from build123d import *

# Parameters (mm, degrees)
SKETCH1_W                 = 23
SKETCH1_H                 = 33
BOSS_EXTRUDE1_DEPTH       = 46
CUT_EXTRUDE1_START        = 12
SKETCH2_W                 = 23
SKETCH2_H                 = 17
CUT_EXTRUDE1_DEPTH        = 26
SKETCH3_R                 = 2.5
CUT_EXTRUDE2_DEPTH        = 6
CUT_EXTRUDE3_START        = -6
SKETCH4_R                 = 2.5
CUT_EXTRUDE3_DEPTH        = 6
CHAMFER1_SIZE             = 6
BOSS_EXTRUDE2_DEPTH       = 26.5
BOSS_EXTRUDE2_DEPTH_BACK  = 23
SKETCH6_W                 = 3
SKETCH6_H                 = 46
F_5_0MM_DOWEL_HOLE1_D     = 5
F_5_0MM_DOWEL_HOLE1_DEPTH = 10
F_5_0MM_DOWEL_HOLE1_TIP   = 1.502151548
SKETCH14_W                = 10
SKETCH14_H                = 10
CUT_EXTRUDE4_DEPTH        = 70.685005561
FILLET1_DEPTH             = 46
FILLET1_START             = 26
FILLET1_2_DEPTH           = 20
FILLET1_3_DEPTH           = 16


with BuildPart() as part:
    # Sketch1 → Boss-Extrude1 (new body)
    with BuildSketch(Plane(origin=(0, 0, 0), x_dir=(1, 0, 0), z_dir=(0, 1, 0))):
        Rectangle(SKETCH1_W, SKETCH1_H)
    extrude(amount=BOSS_EXTRUDE1_DEPTH)

    # Sketch2 → Cut-Extrude1 (cut)
    with BuildSketch(Plane(origin=(0, 0, 0), x_dir=(1, 0, 0), z_dir=(0, 1, 0)).offset(CUT_EXTRUDE1_START)):
        with Locations((0, 8)):
            Rectangle(SKETCH2_W, SKETCH2_H)
    extrude(amount=CUT_EXTRUDE1_DEPTH, mode=Mode.SUBTRACT)

    # Sketch3 → Cut-Extrude2 (cut)
    with BuildSketch(Plane(origin=(0, 46, 0), x_dir=(1, 0, 0), z_dir=(0, 1, 0))):
        with Locations(Location((0, -11.5, 0), (0, 0, 270))):
            Circle(SKETCH3_R)
        with Locations(Location((0, 3.5, 0), (0, 0, 270))):
            Circle(SKETCH3_R)
    extrude(amount=-CUT_EXTRUDE2_DEPTH, mode=Mode.SUBTRACT)

    # Sketch4 → Cut-Extrude3 (cut)
    with BuildSketch(Plane.XZ.offset(CUT_EXTRUDE3_START)):
        with Locations(Location((0, -3.5, 0), (0, 0, 90))):
            Circle(SKETCH4_R)
        with Locations(Location((0, 11.5, 0), (0, 0, 90))):
            Circle(SKETCH4_R)
    extrude(amount=CUT_EXTRUDE3_DEPTH, mode=Mode.SUBTRACT)

    # Chamfer1
    chamfer1_edges = [part.edges().sort_by_distance(p)[0] for p in [
        (11.5, 25, 0.5),
    ]]
    chamfer(chamfer1_edges, length=CHAMFER1_SIZE)

    # Sketch6 → Boss-Extrude2 (add, two sides: drawn at the far end of the back side and taken through both)
    with BuildSketch(Plane(origin=(11.5, 0, 0), x_dir=(0, 0, -1), z_dir=(1, 0, 0)).offset(-BOSS_EXTRUDE2_DEPTH_BACK)):
        with Locations((-18, 23)):
            Rectangle(SKETCH6_W, SKETCH6_H)
    extrude(amount=BOSS_EXTRUDE2_DEPTH + BOSS_EXTRUDE2_DEPTH_BACK)

    # Ø5.0mm Dowel Hole1
    with Locations(Plane(origin=(0, 0, -16.5), x_dir=(-1, 0, 0), z_dir=(0, 0, -1))):
        with Locations((-8, 42), (-8, 8), (8, 8), (8, 42)):
            Hole(F_5_0MM_DOWEL_HOLE1_D / 2, depth=F_5_0MM_DOWEL_HOLE1_DEPTH)
            with Locations((0, 0, -(F_5_0MM_DOWEL_HOLE1_DEPTH + F_5_0MM_DOWEL_HOLE1_TIP / 2))):  # 118° drill point
                Cone(0, F_5_0MM_DOWEL_HOLE1_D / 2, F_5_0MM_DOWEL_HOLE1_TIP, mode=Mode.SUBTRACT)

    # Sketch14 → Cut-Extrude4 (cut, through all)
    with BuildSketch(Plane.XY.offset(19.5)):
        with Locations((23, 21)):
            Rectangle(SKETCH14_W, SKETCH14_H)
    extrude(amount=-CUT_EXTRUDE4_DEPTH, mode=Mode.SUBTRACT)

    # Sketch15 → Cut-Revolve1 (revolve, cut)
    with BuildSketch(Plane(origin=(0, 0, 0), x_dir=(0, 0, -1), z_dir=(1, 0, 0))):
        Polygon((16.5, 46), (13.25, 46), (13.25, 41.999935081), (11.5, 41.999935081), (11.5, 7), (13.25, 7), (13.25, 0), (16.5, 0), align=None)
    revolve(axis=Axis((0, 0, -16.5), (0, 1, 0)), mode=Mode.SUBTRACT)

    # Fillet1: read off the stored shape, not the designer's step
    # Fillet1 outline → Fillet1 (add)
    with BuildSketch(Plane(origin=(0, 0, 0), x_dir=(1, 0, 0), z_dir=(0, 1, 0))):
        with BuildLine():
            Line((18, -16.5), (18, -15.867496998))
            ThreePointArc((18, -15.867496998), (13.284161637, -12.200877126), (11.5, -6.5))
            Line((11.5, -6.5), (11.5, -16.5))
            Line((11.5, -16.5), (18, -16.5))
        make_face()
    extrude(amount=FILLET1_DEPTH)

    # Fillet1 2 outline → Fillet1 2 (add)
    with BuildSketch(Plane(origin=(0, 0, 0), x_dir=(1, 0, 0), z_dir=(0, 1, 0)).offset(FILLET1_START)):
        with BuildLine():
            ThreePointArc((21.5, -16.5), (19.721653855, -16.340603894), (18, -15.867496998))
            Line((18, -15.867496998), (18, -16.5))
            Line((18, -16.5), (21.5, -16.5))
        make_face()
    extrude(amount=FILLET1_2_DEPTH)

    # Fillet1 3 outline → Fillet1 3 (add)
    with BuildSketch(Plane(origin=(0, 0, 0), x_dir=(1, 0, 0), z_dir=(0, 1, 0))):
        with BuildLine():
            ThreePointArc((21.5, -16.5), (19.721653855, -16.340603894), (18, -15.867496998))
            Line((18, -15.867496998), (18, -16.5))
            Line((18, -16.5), (21.5, -16.5))
        make_face()
    extrude(amount=FILLET1_3_DEPTH)


solid = part.part
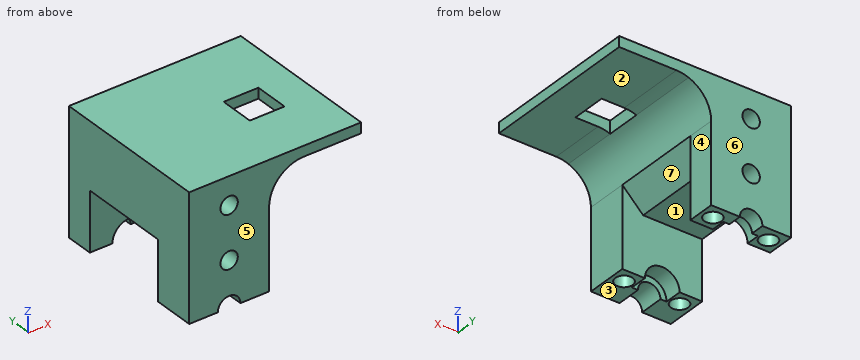
Model file for the job. Use its own axes, mm. Face numbers are marked on the shaded views. A direction names the side the tool comes from. Round coordinates to 2 decimals unless told otherwise and drop trailing zeros. Loops run counter-clockwise (first coordinate to the right, second up) from the corner with the lowest first, then second, coordinate; pieces in that order, holes last. Notation, with made-up numbers: (5, 48.5) - (35, 48.5) arc R21 ccw to (35, 58.5) - close; hole circle Ø4 at (9.5, -19). An arc over 180 degrees is marked (long way). Write each question's results on one line, items separated by ' | '.
(1) Saw through at B-B, the plane x = 25. List the corners of the cut face in (y, z), then the cut area to 3 significant figures.
Answer below:
outline: (0, 16.5) - (16, 16.5) - (16, 19.5) - (0, 19.5) - close; (26, 16.5) - (46, 16.5) - (46, 19.5) - (26, 19.5) - close | area: 108 mm^2
(2) Saw through at C-C, the plane y = 31.5. List the corners of the cut face in (x, z).
Answer below:
outline: (-11.5, 0.5) - (5.5, 0.5) - (11.5, 6.5) arc R10 cw to (21.5, 16.5) - (38, 16.5) - (38, 19.5) - (-11.5, 19.5) - close
(3) Mould opens along Y. For the marked faces 4, 5, 6 and 7 say: released by +Y, released by -Y, zero draft, split by the parting line, or undercut.
Answer below:
face 4: zero draft | face 5: released by -Y | face 6: released by +Y | face 7: undercut
(4) Wall check: L1, parallel to Y at x = 8, z = -9; L2, parallel to X at y = 8, z = -11; L3, parallel to X at y = 40, z = -13. Give the ranges that are in metal, low to high.
Answer below:
L1: y = 0 to 5.5, 10.5 to 12, 38 to 39.5, 44.5 to 46 | L2: x = -11.5 to -10.5, -5.5 to 5.5, 10.5 to 11.5 | L3: x = -11.5 to -9.5, -6.5 to -3.57, 3.57 to 6.5, 9.5 to 11.5
(5) Saw through at A-A, the plane z = -3.5. List the corners of the cut face in (x, y).
Answer below:
outline: (-11.5, 0) - (-2.5, 0) - (-2.5, 6) - (2.5, 6) - (2.5, 0) - (11.5, 0) - (11.5, 12) - (-11.5, 12) - close; (-11.5, 38) - (11.5, 38) - (11.5, 46) - (2.5, 46) - (2.5, 40) - (-2.5, 40) - (-2.5, 46) - (-11.5, 46) - close
(6) Saw through at D-D, the plane x = 0. List the corners of the cut face in (y, z), then the cut area to 3 significant figures.
Answer below:
outline: (0, -13.25) - (7, -13.25) - (7, -11.5) - (12, -11.5) - (12, 0.5) - (38, 0.5) - (38, -11.5) - (42, -11.5) - (42, -13.25) - (46, -13.25) - (46, -6) - (40, -6) - (40, -1) - (46, -1) - (46, 9) - (40, 9) - (40, 14) - (46, 14) - (46, 19.5) - (0, 19.5) - (0, 14) - (6, 14) - (6, 9) - (0, 9) - (0, -1) - (6, -1) - (6, -6) - (0, -6) - close | area: 1,010 mm^2
(7) Pin check, flat tips, straight feed: pin 1 (5 mm diameter, centred on x = 30, y = 24.5, fed in from -Z); pin 2 (9 mm diameter, centred on y = 42.5, z = 0, fed in from +X); pin 3 (4.5 mm diameter, centred on x = -8, y = 42, fed in from -Z). Stop position of each tip, or through.
Answer below:
pin 1: stops at z = 16.5 | pin 2: stops at x = 11.5 | pin 3: stops at z = -6.35
(8) 3-axis set-ups, long thin cutter, end or side, ignore diameter. For the marked faces 1, 2 and 3: which of +Z, -Z, +X, -X, +Y, -Y reach the whole face in a straight line?
Answer below:
face 1: -Z, +X, -X | face 2: -Z, +X, +Y, -Y | face 3: -Z, +X, -X, +Y, -Y
